Here's how the part is built. I have some questions about the finished solid (model axes, mm). Face numbers are marked on the shaded views. A direction names the side the tool comes from. Coordinates: 2 decimals unless noted, no trailing zeros. Loops run counter-clockwise (first coordinate to the right, second up) from the corner with the lowest first, then second, coordinate; pieces in that order, holes last. Notation, with made-up numbers: M 82,-10 L 122,-10 A20 cw 122,16 Z; hole C -5.5,-18.75 d9. An arc over 180 degrees is marked long. Use CSV: the item, a comma, the result in double quotes. Start each with the question number.
Q1. If we section it at A-A (x = 0): Please give me the cut outline in (y, z), and give its area (3 significant figures).
Q2. For pin 1 Ø0.5 at (y, z) = (19, 18.5) entering from +X; pin 2 Ø1.8 at (x, y) = (3.5, 51.61) entering from +Z; pin 3 Ø3 at (x, z) = (5.5, 7.5) entering from +Y, each with a flat end and sliding along its axis, tell me the tip position at first contact or that it passes through.
Q3. If we section it at B-B (y = 26): Please give me the cut outline in (x, z), and give its area (3 significant figures).
Q4. If we section it at C-C (y = 43): Please give me the cut outline in (x, z).
Q5. If we mould it in two halves opening along Z, with no side actions, what happens to the marked faces 3, 4 and 5? For each: +Z half, -Z half, draft (parallel to the pull), parting line (faces both ways), or undercut.
Q6. Which directions (+Z, -Z, +X, -X, +Y, -Y) give clear straight access to the entire face, cutting with the end or side of a thin tool? Please do the marked faces 1 and 2.
Q7. Please list where these lines run through material, in increasing order: probe 1 along Z at (x, y) = (1, 53.5); probe 2 along Y at (x, z) = (-1, -11). Write a range as [from, to].
Q8. If we section it at D-D (z = 15): Please give me the cut outline in (x, y).
from build123d import *

# Parameters (mm, degrees)
ESQUISSE1_W             = 24
ESQUISSE1_H             = 38.58
BOSS_EXTRU_1_DEPTH      = 1.5875
ESQUISSE5_R             = 1
ESQUISSE5_R_2           = 4
BOSS_EXTRU_8_DEPTH      = 1.5875
ESQUISSE8_R             = 1
ESQUISSE8_R_2           = 4
BOSS_EXTRU_10_DEPTH     = 1.5875
ESQUISSE11_R            = 1
ENL_V_MAT_EXTRU_3_DEPTH = 1.5875


with BuildPart() as part:
    # Esquisse1 → Boss.-Extru.1 (new body)
    with BuildSketch(Plane(origin=(0, 0, 0), x_dir=(1, 0, 0), z_dir=(0, 1, 0))):
        Rectangle(ESQUISSE1_W, ESQUISSE1_H)
    extrude(amount=BOSS_EXTRU_1_DEPTH)

    # Esquisse5 → Boss.-Extru.8 (add)
    # profile 1 of 7: a face of its own
    with BuildSketch(Plane.XY.offset(19.29)):
        with BuildLine():
            Line((-9.5, 45.543001341), (-9.5, 1.5875))
            Line((-9.5, 1.5875), (9.5, 1.5875))
            Line((9.5, 1.5875), (9.5, 45.543001341))
            ThreePointArc((9.5, 45.543001341), (0, 55.043001341), (-9.5, 45.543001341))
        make_face()
        with Locations((-3.5, 39.480823515)):
            Circle(ESQUISSE5_R, mode=Mode.SUBTRACT)
        with Locations((-6.062177826, 42.043001341)):
            Circle(ESQUISSE5_R, mode=Mode.SUBTRACT)
        with Locations((-7, 45.543001341)):
            Circle(ESQUISSE5_R, mode=Mode.SUBTRACT)
        with Locations((-6.062177826, 49.043001341)):
            Circle(ESQUISSE5_R, mode=Mode.SUBTRACT)
        with Locations((-3.5, 51.605179168)):
            Circle(ESQUISSE5_R, mode=Mode.SUBTRACT)
        with Locations((0, 38.543001341)):
            Circle(ESQUISSE5_R, mode=Mode.SUBTRACT)
        with Locations((3.5, 39.480823515)):
            Circle(ESQUISSE5_R, mode=Mode.SUBTRACT)
        with Locations((0, 45.543001341)):
            Circle(ESQUISSE5_R_2, mode=Mode.SUBTRACT)
        with Locations((0, 52.543001341)):
            Circle(ESQUISSE5_R, mode=Mode.SUBTRACT)
        with Locations((3.5, 51.605179168)):
            Circle(ESQUISSE5_R, mode=Mode.SUBTRACT)
        with Locations((6.062177826, 42.043001341)):
            Circle(ESQUISSE5_R, mode=Mode.SUBTRACT)
        with Locations((7, 45.543001341)):
            Circle(ESQUISSE5_R, mode=Mode.SUBTRACT)
        with Locations((6.062177826, 49.043001341)):
            Circle(ESQUISSE5_R, mode=Mode.SUBTRACT)
    # profile 2 of 7: a face of its own
    with BuildSketch(Plane.XY.offset(19.29)):
        with Locations((0, 38.543001341)):
            Circle(ESQUISSE5_R)
    # profile 3 of 7: a face of its own
    with BuildSketch(Plane.XY.offset(19.29)):
        with Locations((6.062177826, 42.043001341)):
            Circle(ESQUISSE5_R)
    # profile 4 of 7: a face of its own
    with BuildSketch(Plane.XY.offset(19.29)):
        with Locations((6.062177826, 49.043001341)):
            Circle(ESQUISSE5_R)
    # profile 5 of 7: a face of its own
    with BuildSketch(Plane.XY.offset(19.29)):
        with Locations((-6.062177826, 42.043001341)):
            Circle(ESQUISSE5_R)
    # profile 6 of 7: a face of its own
    with BuildSketch(Plane.XY.offset(19.29)):
        with Locations((-6.062177826, 49.043001341)):
            Circle(ESQUISSE5_R)
    # profile 7 of 7: a face of its own
    with BuildSketch(Plane.XY.offset(19.29)):
        with Locations((0, 52.543001341)):
            Circle(ESQUISSE5_R)
    extrude(amount=-BOSS_EXTRU_8_DEPTH)

    # Esquisse8 → Boss.-Extru.10 (add)
    # profile 1 of 13: a face of its own
    with BuildSketch(Plane(origin=(0, 0, -19.29), x_dir=(-1, 0, 0), z_dir=(0, 0, -1))):
        with BuildLine():
            Line((-9.5, 45.5), (-9.5, 1.5875))
            Line((-9.5, 1.5875), (9.504737636, 1.5875))
            Line((9.504737636, 1.5875), (9.504737636, 45.5))
            ThreePointArc((9.504737636, 45.5), (0.002368818, 55.002368818), (-9.5, 45.5))
        make_face()
        with Locations((-3.497631182, 39.437822174)):
            Circle(ESQUISSE8_R, mode=Mode.SUBTRACT)
        with Locations((-6.059809008, 42)):
            Circle(ESQUISSE8_R, mode=Mode.SUBTRACT)
        with Locations((-6.997631182, 45.5)):
            Circle(ESQUISSE8_R, mode=Mode.SUBTRACT)
        with Locations((-6.059809008, 49)):
            Circle(ESQUISSE8_R, mode=Mode.SUBTRACT)
        with Locations((-3.497631182, 51.562177826)):
            Circle(ESQUISSE8_R, mode=Mode.SUBTRACT)
        with Locations((0.002368818, 38.5)):
            Circle(ESQUISSE8_R, mode=Mode.SUBTRACT)
        with Locations((3.502368818, 39.437822174)):
            Circle(ESQUISSE8_R, mode=Mode.SUBTRACT)
        with Locations((0.002368818, 45.5)):
            Circle(ESQUISSE8_R_2, mode=Mode.SUBTRACT)
        with Locations((0.002368818, 52.5)):
            Circle(ESQUISSE8_R, mode=Mode.SUBTRACT)
        with Locations((3.502368818, 51.562177826)):
            Circle(ESQUISSE8_R, mode=Mode.SUBTRACT)
        with Locations((6.064546644, 42)):
            Circle(ESQUISSE8_R, mode=Mode.SUBTRACT)
        with Locations((7.002368818, 45.5)):
            Circle(ESQUISSE8_R, mode=Mode.SUBTRACT)
        with Locations((6.064546644, 49)):
            Circle(ESQUISSE8_R, mode=Mode.SUBTRACT)
    # profile 2 of 13: a face of its own
    with BuildSketch(Plane(origin=(0, 0, -19.29), x_dir=(-1, 0, 0), z_dir=(0, 0, -1))):
        with Locations((6.064546644, 49)):
            Circle(ESQUISSE8_R)
    # profile 3 of 13: a face of its own
    with BuildSketch(Plane(origin=(0, 0, -19.29), x_dir=(-1, 0, 0), z_dir=(0, 0, -1))):
        with Locations((6.064546644, 42)):
            Circle(ESQUISSE8_R)
    # profile 4 of 13: a face of its own
    with BuildSketch(Plane(origin=(0, 0, -19.29), x_dir=(-1, 0, 0), z_dir=(0, 0, -1))):
        with Locations((0.002368818, 38.5)):
            Circle(ESQUISSE8_R)
    # profile 5 of 13: a face of its own
    with BuildSketch(Plane(origin=(0, 0, -19.29), x_dir=(-1, 0, 0), z_dir=(0, 0, -1))):
        with Locations((-6.059809008, 42)):
            Circle(ESQUISSE8_R)
    # profile 6 of 13: a face of its own
    with BuildSketch(Plane(origin=(0, 0, -19.29), x_dir=(-1, 0, 0), z_dir=(0, 0, -1))):
        with Locations((-6.059809008, 49)):
            Circle(ESQUISSE8_R)
    # profile 7 of 13: a face of its own
    with BuildSketch(Plane(origin=(0, 0, -19.29), x_dir=(-1, 0, 0), z_dir=(0, 0, -1))):
        with Locations((0.002368818, 52.5)):
            Circle(ESQUISSE8_R)
    # profile 8 of 13: a face of its own
    with BuildSketch(Plane(origin=(0, 0, -19.29), x_dir=(-1, 0, 0), z_dir=(0, 0, -1))):
        with Locations((-6.997631182, 45.5)):
            Circle(ESQUISSE8_R)
    # profile 9 of 13: a face of its own
    with BuildSketch(Plane(origin=(0, 0, -19.29), x_dir=(-1, 0, 0), z_dir=(0, 0, -1))):
        with Locations((-3.497631182, 51.562177826)):
            Circle(ESQUISSE8_R)
    # profile 10 of 13: a face of its own
    with BuildSketch(Plane(origin=(0, 0, -19.29), x_dir=(-1, 0, 0), z_dir=(0, 0, -1))):
        with Locations((3.502368818, 51.562177826)):
            Circle(ESQUISSE8_R)
    # profile 11 of 13: a face of its own
    with BuildSketch(Plane(origin=(0, 0, -19.29), x_dir=(-1, 0, 0), z_dir=(0, 0, -1))):
        with Locations((7.002368818, 45.5)):
            Circle(ESQUISSE8_R)
    # profile 12 of 13: a face of its own
    with BuildSketch(Plane(origin=(0, 0, -19.29), x_dir=(-1, 0, 0), z_dir=(0, 0, -1))):
        with Locations((3.502368818, 39.437822174)):
            Circle(ESQUISSE8_R)
    # profile 13 of 13: a face of its own
    with BuildSketch(Plane(origin=(0, 0, -19.29), x_dir=(-1, 0, 0), z_dir=(0, 0, -1))):
        with Locations((-3.497631182, 39.437822174)):
            Circle(ESQUISSE8_R)
    extrude(amount=-BOSS_EXTRU_10_DEPTH)

    # Esquisse11 → Enl_v. mat.-Extru.3 (cut)
    with BuildSketch(Plane(origin=(0, 1.5875, 0), x_dir=(1, 0, 0), z_dir=(0, 1, 0))):
        with Locations(Location((-9, 9, 0), (0, 0, 270))):
            Circle(ESQUISSE11_R)
        with Locations(Location((9, 9, 0), (0, 0, 270))):
            Circle(ESQUISSE11_R)
        with Locations(Location((9, -9, 0), (0, 0, 270))):
            Circle(ESQUISSE11_R)
        with Locations(Location((-9, -9, 0), (0, 0, 270))):
            Circle(ESQUISSE11_R)
    extrude(amount=-ENL_V_MAT_EXTRU_3_DEPTH, mode=Mode.SUBTRACT)


solid = part.part
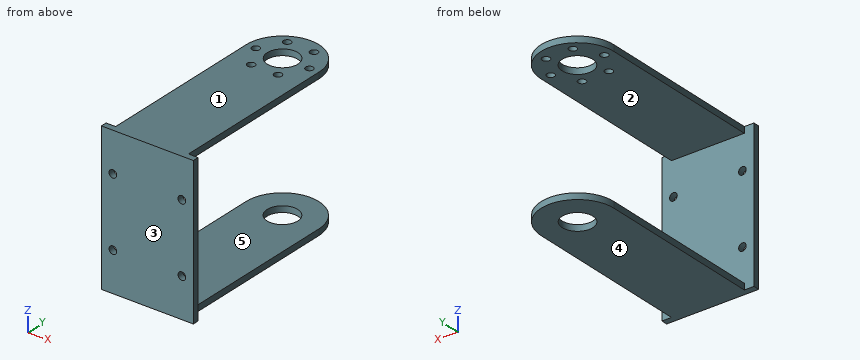
Results below:
1,outline,"M 0,-19.29 L 41.5,-19.29 L 41.5,-17.7 L 1.59,-17.7 L 1.59,17.7 L 41.54,17.7 L 41.54,19.29 L 0,19.29 Z; M 49.5,-19.29 L 55,-19.29 L 55,-17.7 L 49.5,-17.7 Z; M 49.54,17.7 L 55.04,17.7 L 55.04,19.29 L 49.54,19.29 Z"
1,area,"206 mm^2"
2,pin 1,"x = 9.5"
2,pin 2,"z = -17.7"
2,pin 3,"y = 1.59"
3,outline,"M -9.5,-19.29 L 9.5,-19.29 L 9.5,-17.7 L -9.5,-17.7 Z; M -9.5,17.7 L 9.5,17.7 L 9.5,19.29 L -9.5,19.29 Z"
3,area,"60.3 mm^2"
4,outline,"M -9.5,-19.29 L -3.12,-19.29 L -3.12,-17.7 L -9.5,-17.7 Z; M -9.5,17.7 L -3.09,17.7 L -3.09,19.29 L -9.5,19.29 Z; M 3.09,17.7 L 9.5,17.7 L 9.5,19.29 L 3.09,19.29 Z; M 3.12,-19.29 L 9.5,-19.29 L 9.5,-17.7 L 3.12,-17.7 Z"
5,face 3,"draft"
5,face 4,"-Z half"
5,face 5,"undercut"
6,face 1,"+Z, +X, -X, +Y, -Y"
6,face 2,"+X, -X, +Y"
7,probe 1,"[-19.29, -17.7], [17.7, 19.29]"
7,probe 2,"[0, 1.59]"
8,outline,"M -12,0 L 12,0 L 12,1.59 L -12,1.59 Z"
